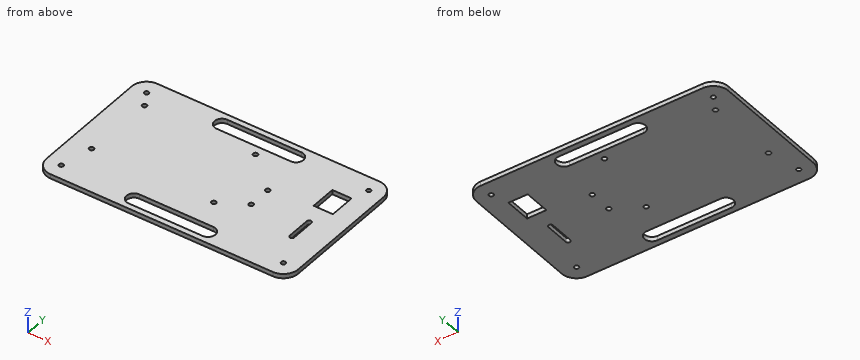
from build123d import *

# Parameters (mm, degrees)
SKETCH1_R           = 1.5
SKETCH1_R_2         = 1.56
SKETCH1_W           = 13
SKETCH1_H           = 17.5
BOSS_EXTRUDE1_DEPTH = 3


with BuildPart() as part:
    # Sketch1 → Boss-Extrude1 (new body)
    with BuildSketch(Plane.XY):
        with BuildLine():
            Line((-75, 50), (75, 50))
            ThreePointArc((75, 50), (82.071067812, 47.071067812), (85, 40))
            Line((85, 40), (85, -40))
            ThreePointArc((85, -40), (82.071067812, -47.071067812), (75, -50))
            Line((75, -50), (-75, -50))
            ThreePointArc((-75, -50), (-82.071067812, -47.071067812), (-85, -40))
            Line((-85, -40), (-85, 40))
            ThreePointArc((-85, 40), (-82.071067812, 47.071067812), (-75, 50))
        make_face()
        with Locations((-75, 40)):
            Circle(SKETCH1_R, mode=Mode.SUBTRACT)
        with Locations((-75, -40)):
            Circle(SKETCH1_R, mode=Mode.SUBTRACT)
        with Locations((75, -40)):
            Circle(SKETCH1_R, mode=Mode.SUBTRACT)
        with Locations((75, 40)):
            Circle(SKETCH1_R, mode=Mode.SUBTRACT)
        with Locations((-69.18, 30)):
            Circle(SKETCH1_R_2, mode=Mode.SUBTRACT)
        with Locations((5.75, 30)):
            Circle(SKETCH1_R_2, mode=Mode.SUBTRACT)
        with Locations((12.37, -18.3)):
            Circle(SKETCH1_R_2, mode=Mode.SUBTRACT)
        with Locations((-70.18, -18.3)):
            Circle(SKETCH1_R_2, mode=Mode.SUBTRACT)
        with Locations((30, 7.78)):
            Circle(SKETCH1_R_2, mode=Mode.SUBTRACT)
        with Locations((30, -7.78)):
            Circle(SKETCH1_R_2, mode=Mode.SUBTRACT)
        with BuildLine():
            Line((-25, 46.257829906), (25, 46.257829906))
            ThreePointArc((25, 46.257829906), (30, 41.257829906), (25, 36.257829906))
            Line((25, 36.257829906), (-25, 36.257829906))
            ThreePointArc((-25, 36.257829906), (-30, 41.257829906), (-25, 46.257829906))
        make_face(mode=Mode.SUBTRACT)
        with BuildLine():
            Line((-25, -46.257829906), (25, -46.257829906))
            ThreePointArc((25, -46.257829906), (30, -41.257829906), (25, -36.257829906))
            Line((25, -36.257829906), (-25, -36.257829906))
            ThreePointArc((-25, -36.257829906), (-30, -41.257829906), (-25, -46.257829906))
        make_face(mode=Mode.SUBTRACT)
        with Locations((65, 20)):
            Rectangle(SKETCH1_W, SKETCH1_H, mode=Mode.SUBTRACT)
        with BuildLine():
            Line((66.5, -1.95), (66.5, -18.05))
            ThreePointArc((66.5, -18.05), (65, -19.55), (63.5, -18.05))
            Line((63.5, -18.05), (63.5, -1.95))
            ThreePointArc((63.5, -1.95), (65, -0.45), (66.5, -1.95))
        make_face(mode=Mode.SUBTRACT)
    extrude(amount=BOSS_EXTRUDE1_DEPTH)


solid = part.part
Geometry check sheet. Reference: the model listing, model coordinates, mm. Coordinates: 2 decimals unless noted, no trailing zeros. Order: outer loops, then holes, each group sorted by start corner. A loop starts at its lowest first (then second) coordinate and runs counter-clockwise, first axis right, second up. Notation, with made-up numbers: (-37, 69.25) - (-1, 69.25) arc R20 cw to (-1, 101.25) - close; hole circle Ø1 at (11.5, -19). An arc over 180 degrees is marked (long way). Answer in a Markdown table with one row per item. Add a question column.
1) Cross-section at C-C, the plane z = 1.6. State how many separate pieces and enclosed holes the cut face has, then the cut area to 3 significant figures.
2) Material ranges on line 1 along Y through (x, z) = (-19, 2.3); line 2 along Y through (x, z) = (-75, 1); line 3 along Y through (x, z) = (5.75, 2.35), recorded low to high. Write a range as [from, to].
3) Cross-section at A-A, the plane y = -13. Record the cut outline in (x, z), then the cut area to 3 significant figures.
4) Cross-section at B-B, the plane x = 0.5. Record the cut outline in (y, z).
Check result:
| question | item | result |
|---|---|---|
| 1 | separate pieces | 1 |
| 1 | enclosed holes | 14 |
| 1 | area | 15,400 mm² |
| 2 | line 1 | y = [-50, -46.26], [-36.26, 36.26], [46.26, 50] |
| 2 | line 2 | y = [-50, -41.5], [-38.5, 38.5], [41.5, 50] |
| 2 | line 3 | y = [-50, -46.26], [-36.26, 28.44], [31.56, 36.26], [46.26, 50] |
| 3 | outline | (-85, 0) - (63.5, 0) - (63.5, 3) - (-85, 3) - close; (66.5, 0) - (85, 0) - (85, 3) - (66.5, 3) - close |
| 3 | area | 501 mm² |
| 4 | outline | (-50, 0) - (-46.26, 0) - (-46.26, 3) - (-50, 3) - close; (-36.26, 0) - (36.26, 0) - (36.26, 3) - (-36.26, 3) - close; (46.26, 0) - (50, 0) - (50, 3) - (46.26, 3) - close |
